from build123d import *

# Parameters (mm, degrees)
BOSS_EXTRU_1_DEPTH           = 3
BOSS_EXTRU_2_DEPTH           = 2
BOSS_EXTRU_3_START           = 2
BOSS_EXTRU_3_DEPTH           = 2
ENL_V_MAT_EXTRU_1_DEPTH      = 12.090536506
ENL_V_MAT_EXTRU_1_DEPTH_BACK = 12.090536506
ESQUISSE5_W                  = 14
ESQUISSE5_H                  = 2.4
ENL_V_MAT_EXTRU_2_DEPTH      = 2


with BuildPart() as part:
    # Esquisse1 → Boss.-Extru.1 (new body)
    with BuildSketch(Plane.XY):
        with BuildLine():
            Line((-5, 0), (-5, 7))
            Line((-5, 7), (5, 7))
            Line((5, 7), (5, 0))
            ThreePointArc((5, 0), (0, -5), (-5, 0))
        make_face()
    extrude(amount=BOSS_EXTRU_1_DEPTH)

    # Esquisse2 → Boss.-Extru.2 (add)
    with BuildSketch(Plane.XY):
        with BuildLine():
            Line((-7, 7), (7, 7))
            Line((7, 7), (7, 0))
            ThreePointArc((7, 0), (0, -7), (-7, 0))
            Line((-7, 0), (-7, 7))
        make_face()
    extrude(amount=-BOSS_EXTRU_2_DEPTH)

    # Esquisse3 → Boss.-Extru.3 (add)
    with BuildSketch(Plane.XY.offset(3).offset(BOSS_EXTRU_3_START)):
        with BuildLine():
            Line((7, 7), (-7, 7))
            Line((-7, 7), (-7, 0))
            ThreePointArc((-7, 0), (0, -7), (7, 0))
            Line((7, 0), (7, 7))
        make_face()
    extrude(amount=-BOSS_EXTRU_3_DEPTH)

    # Esquisse4 → Enlèv. mat.-Extru.1 (cut, two sides: drawn at the far end of the back side and taken through both)
    with BuildSketch(Plane.XY.offset(-ENL_V_MAT_EXTRU_1_DEPTH_BACK)):
        with BuildLine():
            ThreePointArc((0.935064935, -1.635355415), (3.65, 0), (0.935064935, 1.635355415))
            ThreePointArc((0.935064935, 1.635355415), (0, 1.403307215), (-0.935064935, 1.635355415))
            ThreePointArc((-0.935064935, 1.635355415), (-3.65, 0), (-0.935064935, -1.635355415))
            ThreePointArc((-0.935064935, -1.635355415), (0, -1.403307215), (0.935064935, -1.635355415))
        make_face()
    extrude(amount=ENL_V_MAT_EXTRU_1_DEPTH + ENL_V_MAT_EXTRU_1_DEPTH_BACK, mode=Mode.SUBTRACT)

    # Esquisse5 → Enlèv. mat.-Extru.2 (cut)
    with BuildSketch(Plane(origin=(0, 0, -2), x_dir=(-1, 0, 0), z_dir=(0, 0, -1))):
        with Locations((0, 5.8)):
            Rectangle(ESQUISSE5_W, ESQUISSE5_H)
    extrude(amount=-ENL_V_MAT_EXTRU_2_DEPTH, mode=Mode.SUBTRACT)


solid = part.part
Could you check a few things on this model? Use its own coordinates, in mm. A direction names the side the tool comes from. Give positions to 0.01 mm unless a question says otherwise; leave off trailing zeros. Order: outer loops, then holes, each group sorted by start corner. A loop starts at its lowest first (then second) coordinate and runs counter-clockwise, first axis right, second up. Notation, with made-up numbers: (-24, 54) - (0, 54) arc R31 ccw to (0, 91) - close; hole circle Ø6 at (1.5, 41). An arc over 180 degrees is marked (long way). Return JSON: item names as keys, results as strings. Group by question number.
Q1. Suppose I cut it at B-B, the plane z = 3.5. Please give me the cut outline in (x, y), and give its area (3 significant figures).
Q2. Which directions (+Z, -Z, +X, -X, +Y, -Y) give clear straight access to the entire face, cutting with the end or side of a thin tool? Please do faces 1 (the face through (0, 4.6, -1)), 2 (the face through (-5, 3, 1)), 3 (the face through (-0.014, -1.403, 1.451)), 4 (the face through (2, -5, 3)).
Q3. Suppose I cut it at D-D, the plane y = -1. Please give me the cut outline in (x, z), and give its area (3 significant figures).
Q4. Suppose I cut it at C-C, the plane y = 3.5. Please give me the cut outline in (x, z).
Q5. Suppose I cut it at A-A, the plane x = 0. Please give me the cut outline in (y, z), and give its area (3 significant figures).
Q6. Thinking about a two-plate mould opening in X: for faces 5 (the face through (0, -7, -1)), 6 (the face through (-7, 4, 4)), 7 (the face through (0.014, 1.403, 1.451)), 8 (the face through (1.07, -5.04, 0)), which applies, pulls with the +X half, pulls with the -X half, needs draft (parallel to the pull), parting line crosses it, or undercut?
Q7. Will these pins go through, and if not, where does the flat tip stop? pin 1 Ø0.7 at (x, y) = (-1.5, 6) entering from -Z; pin 2 Ø1.5 at (x, z) = (-1, 4.5) entering from -Y; pin 3 Ø1.6 at (x, z) = (2.5, -1.5) entering from +Y.
Q8. Please list where these lines run through material, in increasing order: line 1 along Z through (x, y) = (5.75, 2); line 2 along Z through (x, y) = (6.25, 5.75); line 3 along Y through (x, z) = (-1.25, 4.75). Write a range as [from, to].
Resolved:
{
 "1": {"outline": "(-7, 0) arc R7 ccw to (7, 0) - (7, 7) - (-7, 7) - close; hole (-0.94, -1.64) arc R2 cw to (0.94, -1.64) arc R1.85 ccw (long way) to (0.94, 1.64) arc R2 cw to (-0.94, 1.64) arc R1.85 ccw (long way) to start", "area": "153 mm2"},
 "2": {"face 1": "-Z, +X, -X, +Y", "face 2": "-X, +Y, -Y", "face 3": "+Z, -Z", "face 4": "-Y"},
 "3": {"outline": "(-6.93, -2) - (-3.36, -2) - (-3.36, 5) - (-6.93, 5) - (-6.93, 3) - (-4.9, 3) - (-4.9, 0) - (-6.93, 0) - close; (3.36, -2) - (6.93, -2) - (6.93, 0) - (4.9, 0) - (4.9, 3) - (6.93, 3) - (6.93, 5) - (3.36, 5) - close", "area": "37.8 mm2"},
 "4": {"outline": "(-7, -2) - (7, -2) - (7, 0) - (5, 0) - (5, 3) - (7, 3) - (7, 5) - (-7, 5) - (-7, 3) - (-5, 3) - (-5, 0) - (-7, 0) - close"},
 "5": {"outline": "(-7, -2) - (-1.4, -2) - (-1.4, 5) - (-7, 5) - (-7, 3) - (-5, 3) - (-5, 0) - (-7, 0) - close; (1.4, -2) - (4.6, -2) - (4.6, 0) - (7, 0) - (7, 5) - (1.4, 5) - close", "area": "67.6 mm2"},
 "6": {"face 5": "parting line crosses it", "face 6": "pulls with the -X half", "face 7": "undercut", "face 8": "needs draft"},
 "7": {"pin 1": "stops at z = 0", "pin 2": "stops at y = -7", "pin 3": "stops at y = 4.6"},
 "8": {"line 1": "z = [-2, 0], [3, 5]", "line 2": "z = [3, 5]", "line 3": "y = [-6.89, -1.77], [1.77, 7]"}
}
